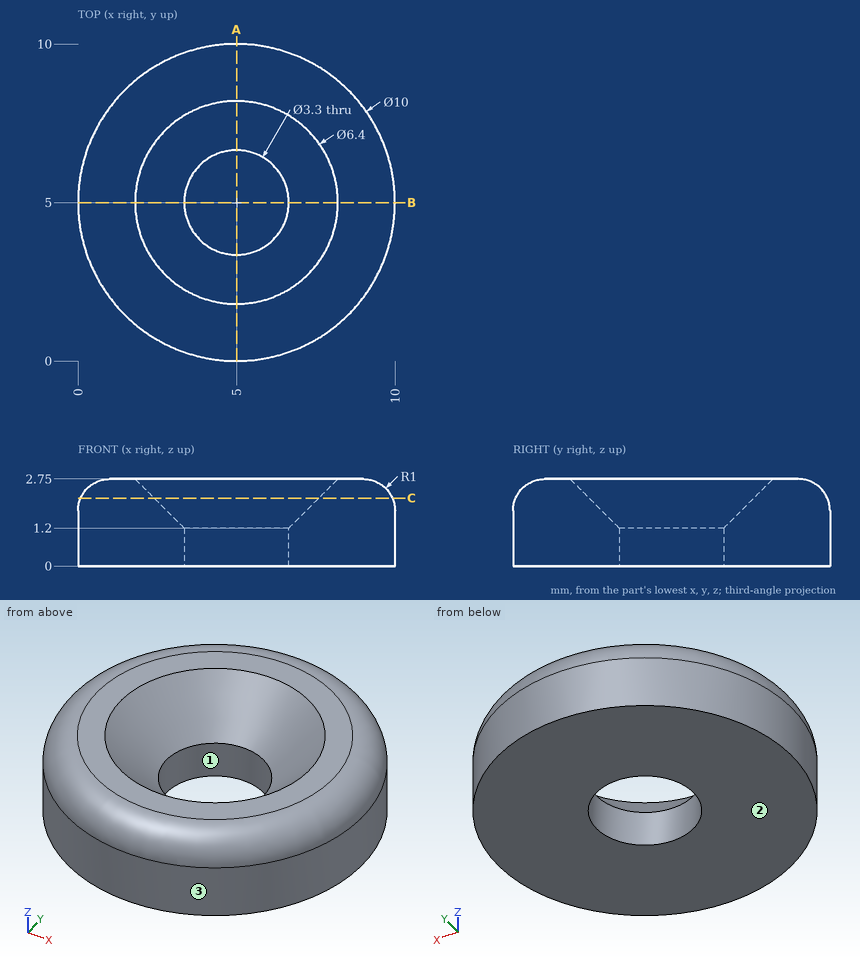
Design review of the part shown in the three views and the two pictorial views. Dimensions are in mm from the part's minimum x, y and z. Coordinates: 2 decimals unless noted, no trailing zeros. Loops run counter-clockwise (first coordinate to the right, second up) from the corner with the lowest first, then second, coordinate; pieces in that order, holes last. Notation, with made-up numbers: (80, -29) -> (117, -29) arc R27 cw to (117, -10) -> close; hole circle Ø8 at (-20.5, 10.25). An arc over 180 degrees is marked (long way). Answer as CSV lines item,"result".
Item 1: Insertion check: pin 1 (6 mm diameter, centred on x = 6.5, y = 8, fed in from -Z); pin 2 (1 mm diameter, centred on y = 7, z = 1, fed in from +X); pin 3 (1 mm diameter, centred on y = 4, z = 1, fed in from -X). Each pin has a flat end and moves straight along its axis. Give the tip position at first contact, or say it passes through.
Results below:
pin 1,"stops at z = 0"
pin 2,"stops at x = 9.77"
pin 3,"stops at x = 0.03"
Item 2: For L1, parallel to Y at x = 5, z = 0.45; L2, parallel to X at y = 5.5, z = 1.1; L3, parallel to Y at x = 6.75, z = 2.6, list the stretches that pass through material, from the lowest coordinate up.
Results below:
L1,"y = 0 to 3.35, 6.65 to 10"
L2,"x = 0.03 to 3.43, 6.57 to 9.97"
L3,"y = 0.83 to 2.5, 7.5 to 9.17"
Item 3: Take a section at C-C, the plane z = 2.15. State the section outline as (x, y) points, and give its area (3 significant figures).
Results below:
outline,"circle Ø9.83 at (5, 5); hole circle Ø5.2 at (5, 5)"
area,"54.7 mm2"
Item 4: Draft analysis for pull direction Y (two halves, no side actions). For the marked faces 1, 2 and 3, state which applies: +Y half, -Y half, draft (parallel to the pull), parting line (faces both ways), or undercut.
Results below:
face 1,"undercut"
face 2,"draft"
face 3,"parting line"
Item 5: Take a section at A-A, the plane x = 5. State the section outline as (y, z) points.
Results below:
outline,"(0, 0) -> (3.35, 0) -> (3.35, 1.2) -> (1.8, 2.75) -> (1, 2.75) arc R1 ccw to (0, 1.75) -> close; (6.65, 0) -> (10, 0) -> (10, 1.75) arc R1 ccw to (9, 2.75) -> (8.2, 2.75) -> (6.65, 1.2) -> close"
